CAD build for the part. Positions are in the model's coordinates, mm. Face numbers are marked on the shaded views. A direction names the side the tool comes from. Round coordinates to 2 decimals unless told otherwise and drop trailing zeros. Order: outer loops, then holes, each group sorted by start corner. A loop starts at its lowest first (then second) coordinate and runs counter-clockwise, first axis right, second up. Notation, with made-up numbers: (1, 84.5) -> (56, 84.5) arc R11 ccw to (56, 94.5) -> close; hole circle Ø4 at (31.5, 31.25). An arc over 180 degrees is marked (long way). Return JSON: item names as keys, results as strings. Group by question number.
Q1. Cut at C-C (z = 2.55). Write the cut outline in (x, y), then the cut area to 3 significant figures.
Q2. Flat gauge pins, fed straight in: pin 1 (1.1 mm diameter, centred on y = -13.5, z = 0.5, fed in from +X); pin 2 (0.8 mm diameter, centred on y = 0, z = 0.5, fed in from -X); pin 3 (6 mm diameter, centred on x = 89.5, y = 0.5, fed in from +Z). Where does each tip first touch, or does it go through?
Q3. Cut at B-B (y = -15). Write the cut outline in (x, z).
Q4. Mould opens along Y. For the marked faces 1, 2, 3 and 4 say: +Y half, -Y half, draft (parallel to the pull), parting line (faces both ways), or undercut.
Q5. Probe line 1 along X through (y, z) = (-15.25, 2.2); line 2 along Y through (x, z) = (109, 3.4); line 3 along X through (y, z) = (1.75, 3.75). List the from-to ranges inside material, lowest first.
Q6. Cut at D-D (y = -10). Write the cut outline in (x, z).
Q7. Which spindle directions (+Z, -Z, +X, -X, +Y, -Y) get a long thin tool onto all of the face, cutting with end or side? Do the marked faces 5, 6 and 7. Say none if no direction does.
Q8. Cut at A-A (x = 92.5). Write the cut outline in (y, z).
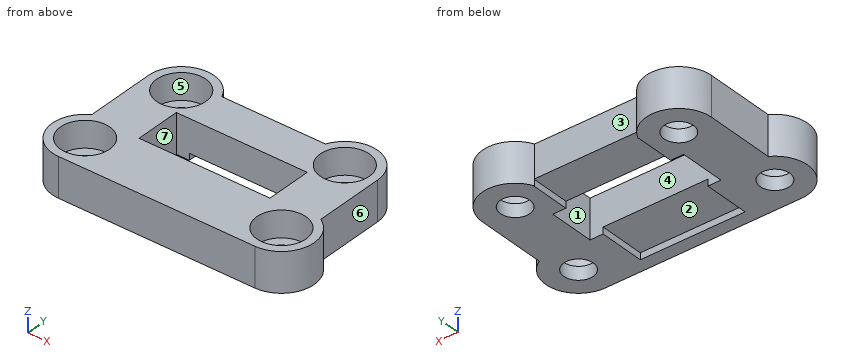
from build123d import *

# Parameters (mm, degrees)
SKETCH155_W         = 20
SKETCH155_H         = 7
PAD067_DEPTH        = 6
HOLE009_D           = 4.5
HOLE009_DEPTH       = 25
HOLE009_CBORE_D     = 7.5
HOLE009_CBORE_DEPTH = 4
SKETCH275_W         = 16
SKETCH275_H         = 20
POCKET114_DEPTH     = 1


with BuildPart() as part:
    # Sketch155 → Pad067 (new body)
    with BuildSketch(Plane.XY):
        with BuildLine():
            Line((-7.917424, 2), (7.917424, 2))
            ThreePointArc((17.5, 0), (13.521548, 4.894532), (7.917424, 2))
            Line((17.5, -10.669873), (17.5, 0))
            ThreePointArc((15, -20), (19.829629, -16.294095), (17.5, -10.669873))
            Line((-14.999993, -20), (15, -20))
            ThreePointArc((-17.5, -10.669873), (-19.829628, -16.294099), (-14.999993, -20))
            Line((-17.5, -10.669873), (-17.5, 0))
            ThreePointArc((-7.917424, 2), (-13.521548, 4.894532), (-17.5, 0))
        make_face()
        with Locations((0, -7.5)):
            Rectangle(SKETCH155_W, SKETCH155_H, mode=Mode.SUBTRACT)
    extrude(amount=PAD067_DEPTH)

    # Hole009
    with Locations(Plane.XY.offset(6)):
        with Locations((-12.5, 0), (12.5, 0), (15, -15), (-15, -15)):
            CounterBoreHole(HOLE009_D / 2, HOLE009_CBORE_D / 2, HOLE009_CBORE_DEPTH, depth=HOLE009_DEPTH)

    # Sketch275 (on Face4 of Hole009) → Pocket114 (cut)
    with BuildSketch(Plane(origin=(0, 0, 0), x_dir=(1, 0, 0), z_dir=(0, 0, -1))):
        with Locations((0, 8)):
            Rectangle(SKETCH275_W, SKETCH275_H)
    extrude(amount=-POCKET114_DEPTH, mode=Mode.SUBTRACT)


with BuildPart() as part_1:
    # Body019 placement: moved
    add(part.part.moved(Location((102, 0, 0))))


solid = part_1.part
Solution:
{
 "1": {"outline": "(84.5, -10.67) arc R5 ccw to (87, -20) -> (117, -20) arc R5 ccw to (119.5, -10.67) -> (119.5, 0) arc R5 ccw to (109.92, 2) -> (94.08, 2) arc R5 ccw to (84.5, 0) -> close; hole circle Ø7.5 at (87, -15); hole circle Ø7.5 at (89.5, 0); hole (92, -11) -> (112, -11) -> (112, -4) -> (92, -4) -> close; hole circle Ø7.5 at (114.5, 0); hole circle Ø7.5 at (117, -15)", "area": "522 mm²"},
 "2": {"pin 1": "stops at x = 121.91", "pin 2": "stops at x = 84.5", "pin 3": "stops at z = 2"},
 "3": {"outline": "(82, 0) -> (84.75, 0) -> (84.75, 2) -> (83.25, 2) -> (83.25, 6) -> (82, 6) -> close; (89.25, 0) -> (94, 0) -> (94, 1) -> (110, 1) -> (110, 0) -> (114.75, 0) -> (114.75, 2) -> (113.25, 2) -> (113.25, 6) -> (90.75, 6) -> (90.75, 2) -> (89.25, 2) -> close; (119.25, 0) -> (122, 0) -> (122, 6) -> (120.75, 6) -> (120.75, 2) -> (119.25, 2) -> close"},
 "4": {"face 1": "undercut", "face 2": "draft", "face 3": "+Y half", "face 4": "undercut"},
 "5": {"line 1": "x = 82.01 to 83.26, 90.74 to 113.26, 120.74 to 121.99", "line 2": "y = -20 to -11, -4 to 2", "line 3": "x = 84.82 to 86.18, 92.82 to 111.18, 117.82 to 119.18"},
 "6": {"outline": "(84.5, 0) -> (92, 0) -> (92, 6) -> (84.5, 6) -> close; (112, 0) -> (119.5, 0) -> (119.5, 6) -> (112, 6) -> close"},
 "7": {"face 5": "+Z", "face 6": "+Z, -Z, +X, +Y", "face 7": "+Z, -Z"},
 "8": {"outline": "(-20, 0) -> (-11, 0) -> (-11, 6) -> (-20, 6) -> close; (-4, 0) -> (4, 0) -> (4, 6) -> (2.25, 6) -> (2.25, 2) -> (-2.25, 2) -> (-2.25, 6) -> (-4, 6) -> close"}
}
